from build123d import *

# Parameters (mm, degrees)
SKETCH_1_W          = 65
SKETCH_1_H          = 30
EXTRUDE_1_DEPTH     = 0.85
FILLET_1_R          = 3.5
HOLE_WIZARD_M2_1_D  = 2.7
SKETCH_6_R          = 0.5
SKETCH_6_R_2        = 1
CUT_EXTRUDE_1_DEPTH = 67.971803768


with BuildPart() as part:
    # 草图1 → 凸台-拉伸1 (new body)
    with BuildSketch(Plane.XY):
        with Locations((29, -11.5)):
            Rectangle(SKETCH_1_W, SKETCH_1_H)
    extrude(amount=EXTRUDE_1_DEPTH)

    # 圆角1
    fillet_1_edges = [part.edges().sort_by_distance(p)[0] for p in [
        (-3.5, 3.5, 0.425),
        (61.5, 3.5, 0.425),
        (61.5, -26.5, 0.425),
        (-3.5, -26.5, 0.425),
    ]]
    fillet(fillet_1_edges, radius=FILLET_1_R)

    # M2 间隙孔1 (through all)
    with Locations(Plane.XY.offset(0.85)):
        with Locations((0, 0), (58, 0), (58, -23), (0, -23)):
            Hole(HOLE_WIZARD_M2_1_D / 2)

    # 草图6 → 切除-拉伸1 (cut, through all)
    with BuildSketch(Plane(origin=(0, 0, 0), x_dir=(-1, 0, 0), z_dir=(0, 0, -1))):
        with Locations((-4.85, 1.3)):
            Circle(SKETCH_6_R)
        with Locations((-4.85, -1.25)):
            Circle(SKETCH_6_R)
        with Locations((-7.4, -1.25)):
            Circle(SKETCH_6_R)
        with Locations((-7.4, 1.3)):
            Circle(SKETCH_6_R)
        with Locations((-9.95, 1.3)):
            Circle(SKETCH_6_R)
        with Locations((-9.95, -1.25)):
            Circle(SKETCH_6_R)
        with Locations((-12.5, -1.25)):
            Circle(SKETCH_6_R)
        with Locations((-12.5, 1.3)):
            Circle(SKETCH_6_R)
        with Locations((-15.05, 1.3)):
            Circle(SKETCH_6_R)
        with Locations((-15.05, -1.25)):
            Circle(SKETCH_6_R)
        with Locations((-17.6, -1.25)):
            Circle(SKETCH_6_R)
        with Locations((-17.6, 1.3)):
            Circle(SKETCH_6_R)
        with Locations((-20.15, 1.3)):
            Circle(SKETCH_6_R)
        with Locations((-20.15, -1.25)):
            Circle(SKETCH_6_R)
        with Locations((-22.7, -1.25)):
            Circle(SKETCH_6_R)
        with Locations((-22.7, 1.3)):
            Circle(SKETCH_6_R)
        with Locations((-25.25, 1.3)):
            Circle(SKETCH_6_R)
        with Locations((-25.25, -1.25)):
            Circle(SKETCH_6_R)
        with Locations((-27.8, -1.25)):
            Circle(SKETCH_6_R)
        with Locations((-27.8, 1.3)):
            Circle(SKETCH_6_R)
        with Locations((-30.35, 1.3)):
            Circle(SKETCH_6_R)
        with Locations((-30.35, -1.25)):
            Circle(SKETCH_6_R)
        with Locations((-32.9, -1.25)):
            Circle(SKETCH_6_R)
        with Locations((-32.9, 1.3)):
            Circle(SKETCH_6_R)
        with Locations((-35.45, 1.3)):
            Circle(SKETCH_6_R)
        with Locations((-35.45, -1.25)):
            Circle(SKETCH_6_R)
        with Locations((-38, -1.25)):
            Circle(SKETCH_6_R)
        with Locations((-38, 1.3)):
            Circle(SKETCH_6_R)
        with Locations((-40.55, 1.3)):
            Circle(SKETCH_6_R)
        with Locations((-40.55, -1.25)):
            Circle(SKETCH_6_R)
        with Locations((-43.1, -1.25)):
            Circle(SKETCH_6_R)
        with Locations((-43.1, 1.3)):
            Circle(SKETCH_6_R)
        with Locations((-45.65, 1.3)):
            Circle(SKETCH_6_R)
        with Locations((-45.65, -1.25)):
            Circle(SKETCH_6_R)
        with Locations((-48.2, -1.25)):
            Circle(SKETCH_6_R)
        with Locations((-48.2, 1.3)):
            Circle(SKETCH_6_R)
        with Locations((-50.75, 1.3)):
            Circle(SKETCH_6_R)
        with Locations((-50.75, -1.25)):
            Circle(SKETCH_6_R)
        with Locations((-53.3, -1.25)):
            Circle(SKETCH_6_R)
        with Locations((-53.3, 1.3)):
            Circle(SKETCH_6_R)
        with Locations((-6.125, 0.025)):
            Circle(SKETCH_6_R_2)
        with Locations((-52.025, 0.025)):
            Circle(SKETCH_6_R_2)
    extrude(amount=-CUT_EXTRUDE_1_DEPTH, mode=Mode.SUBTRACT)


solid = part.part
Source: CAD feature listing. Evaluate the final solid. Frame: model axes, mm. Coordinates: 2 decimals unless noted, no trailing zeros.
Item 1: Cut plane A-A (z = 0.7). Count the separate pieces of the cut face and the enclosed holes in it, plus the area to 3 significant figures.
Output values:
separate pieces: 1
enclosed holes: 46
area: 1,880 mm2
Item 2: Pull-direction query (X, two-part tool) for faces 1 (the face through (0.29, -1.32, 0.42)), 2 (the face through (29, -11, 0)), 3 (the face through (-2.5, -25.45, 0.43)); classes: pulls with the +X half, pulls with the -X half, needs draft (parallel to the pull), parting line crosses it, or undercut.
Output values:
face 1: undercut
face 2: needs draft
face 3: pulls with the -X half
Item 3: Material intervals for line 1 (Y direction, x = 58, z = 0.2); line 2 (Y direction, x = 25.25, z = 0.35), sorted ascending.
Output values:
line 1: y = -26.5 to -24.35, -21.65 to -1.35, 1.35 to 3.5
line 2: y = -26.5 to -1.75, -0.75 to 0.8, 1.8 to 3.5
